from build123d import *

# Parameters (mm, degrees)
F1_DEPTH = 38.1
F3_DEPTH = 152.4


with BuildPart() as f1:
    # F0 (on Right) → F1 (new body, symmetric)
    with BuildSketch(Plane.YZ):
        with BuildLine():
            ThreePointArc((33.2424010234, 703.5666301797), (75.487634561, 624.6049517374), (13.4725780266, 560.0004690593))
            Line((13.4725780266, 560.0004690593), (-558.8, 457.2))
            Line((-558.8, 457.2), (-914.4, 457.2))
            Line((-914.4, 457.2), (-914.4, 0))
            Line((-914.4, 0), (762, 0))
            Line((762, 0), (762, 1752.6))
            Line((762, 1752.6), (0, 1752.6))
            Line((0, 1752.6), (-558.8, 1295.4))
            Line((-558.8, 1295.4), (-914.4, 1295.4))
            Line((-914.4, 1295.4), (-914.4, 990.6))
            Line((-914.4, 990.6), (-558.8, 990.6))
            Line((-558.8, 990.6), (33.2424010234, 703.5666301797))
        make_face()
    extrude(amount=F1_DEPTH, both=True)

    # F2 (on Right) → F3 (join, symmetric)
    with BuildSketch(Plane.YZ):
        with BuildLine():
            Line((-558.8, 990.6), (33.2424010234, 703.5666301797))
            ThreePointArc((33.2424010234, 703.5666301797), (75.487634561, 624.6049517374), (13.4725780266, 560.0004690593))
            Line((13.4725780266, 560.0004690593), (-558.8, 457.2))
            Line((-558.8, 457.2), (-914.4, 457.2))
            Line((-914.4, 457.2), (-914.4, 0))
            Line((-914.4, 0), (762, 0))
            Line((762, 0), (762, 1752.6))
            Line((762, 1752.6), (0, 1752.6))
            Line((0, 1752.6), (-558.8, 1295.4))
            Line((-558.8, 1295.4), (-914.4, 1295.4))
            Line((-914.4, 1295.4), (-914.4, 990.6))
            Line((-914.4, 990.6), (-558.8, 990.6))
        make_face()
        with BuildLine():
            Line((698.5, 1689.1), (698.5, 63.5))
            Line((698.5, 63.5), (-850.9, 63.5))
            Line((-850.9, 63.5), (-850.9, 393.7))
            Line((-850.9, 393.7), (-553.1418560933, 393.7))
            Line((-553.1418560933, 393.7), (24.699726382, 497.5008599421))
            ThreePointArc((24.699726382, 497.5008599421), (138.3939966952, 615.9424115186), (60.9444018763, 760.7054886627))
            Line((60.9444018763, 760.7054886627), (-544.2186530254, 1054.1))
            Line((-544.2186530254, 1054.1), (-850.9, 1054.1))
            Line((-850.9, 1054.1), (-850.9, 1231.9))
            Line((-850.9, 1231.9), (-536.1328254861, 1231.9))
            Line((-536.1328254861, 1231.9), (22.6671745139, 1689.1))
            Line((22.6671745139, 1689.1), (698.5, 1689.1))
        make_face(mode=Mode.SUBTRACT)
    extrude(amount=F3_DEPTH, both=True)


solid = f1.part
Read the model definition and answer for the solid it produces. Units are mm, in the model's axes. A direction names the side the tool comes from. Coordinates: 2 decimals unless noted, no trailing zeros. Order: outer loops, then holes, each group sorted by start corner. A loop starts at its lowest first (then second) coordinate and runs counter-clockwise, first axis right, second up. Notation, with made-up numbers: M 83,62.5 L 125,62.5 A29 ccw 125,84.5 Z; hole C 65.25,28 d2. An arc over 180 degrees is marked long. Put each result on its own line as item: value. Start each with the question number.
Item 1: The mould has two halves that part along Z. Classify faces 1 (the face through (2, -734, 1295.4)), 2 (the face through (2, -88, 0)), 3 (the face through (2, -734, 457.2)): +Z half, -Z half, draft (parallel to the pull), parting line (faces both ways), or undercut.
Item 2: For faces 4 (the face through (96.05, -260.644, 1457.3)), 5 (the face through (2, -739, 990.6)), 6 (the face through (-94.45, 138.037, 613.512)), determine the directions among +Z, -Z, +X, -X, +Y, -Y from which every point of the face is accessible in a straight line to the end or side of a thin tool.
Item 3: Given pin 1 Ø5 at (x, y) = (-51.5, -60) entering from +Z; pin 2 Ø12 at (x, z) = (-112.5, 1554) entering from -Y; pin 3 Ø2 at (x, y) = (-0.5, -468.5) entering from +Z, each flat-ended and moving along its own axis, determine where each tip first touches the part or whether it passes through.
Item 4: Section C-C, the plane y = 477.5 is taken. Determine the outline of the cut face in (x, z), plus the area to 3 significant figures.
Item 5: Section D-D, the plane y = -188 is taken. Determine the outline of the cut face in (x, z).
Item 6: Section B-B, the plane x = -9.5 is taken. Determine the outline of the cut face in (y, z), plus the area to 3 significant figures.
Item 7: Section A-A, the plane y = -741 is taken. Determine the outline of the cut face in (x, z), plus the area to 3 significant figures.
Item 8: Consider probe 1 along Z at (x, y) = (-44, 665.5); probe 2 along Y at (x, z) = (59, 375); probe 3 along Y at (x, z) = (-106.5, 640). Determine where each line is inside the solid, lowest interval first. Write a range as [from, to].
Computed:
1. face 1: +Z half
1. face 2: -Z half
1. face 3: undercut
2. face 4: +X
2. face 5: +X, -X, -Y
2. face 6: -X
3. pin 1: stops at z = 1705.55
3. pin 2: stops at y = -250.07
3. pin 3: stops at z = 1370.1
4. outline: M -152.4,0 L 152.4,0 L 152.4,63.5 L 38.1,63.5 L 38.1,1689.1 L 152.4,1689.1 L 152.4,1752.6 L -152.4,1752.6 L -152.4,1689.1 L -38.1,1689.1 L -38.1,63.5 L -152.4,63.5 Z
4. area: 163,000 mm2
5. outline: M -152.4,0 L 152.4,0 L 152.4,63.5 L 38.1,63.5 L 38.1,459.29 L 152.4,459.29 L 152.4,523.81 L -152.4,523.81 L -152.4,459.29 L -38.1,459.29 L -38.1,63.5 L -152.4,63.5 Z; M -152.4,810.83 L 152.4,810.83 L 152.4,881.4 L 38.1,881.4 L 38.1,1516.74 L 152.4,1516.74 L 152.4,1598.78 L -152.4,1598.78 L -152.4,1516.74 L -38.1,1516.74 L -38.1,881.4 L -152.4,881.4 Z
6. outline: M -914.4,0 L 762,0 L 762,1752.6 L 0,1752.6 L -558.8,1295.4 L -914.4,1295.4 L -914.4,990.6 L -558.8,990.6 L 33.24,703.57 A76.2 cw 13.47,560 L -558.8,457.2 L -914.4,457.2 Z
6. area: 2,250,000 mm2
7. outline: M -152.4,0 L 152.4,0 L 152.4,63.5 L 38.1,63.5 L 38.1,393.7 L 152.4,393.7 L 152.4,457.2 L -152.4,457.2 L -152.4,393.7 L -38.1,393.7 L -38.1,63.5 L -152.4,63.5 Z; M -152.4,990.6 L 152.4,990.6 L 152.4,1054.1 L 38.1,1054.1 L 38.1,1231.9 L 152.4,1231.9 L 152.4,1295.4 L -152.4,1295.4 L -152.4,1231.9 L -38.1,1231.9 L -38.1,1054.1 L -152.4,1054.1 Z
7. area: 116,000 mm2
8. probe 1: z = [0, 63.5], [1689.1, 1752.6]
8. probe 2: y = [-914.4, -850.9], [698.5, 762]
8. probe 3: y = [76.04, 139.61], [698.5, 762]
